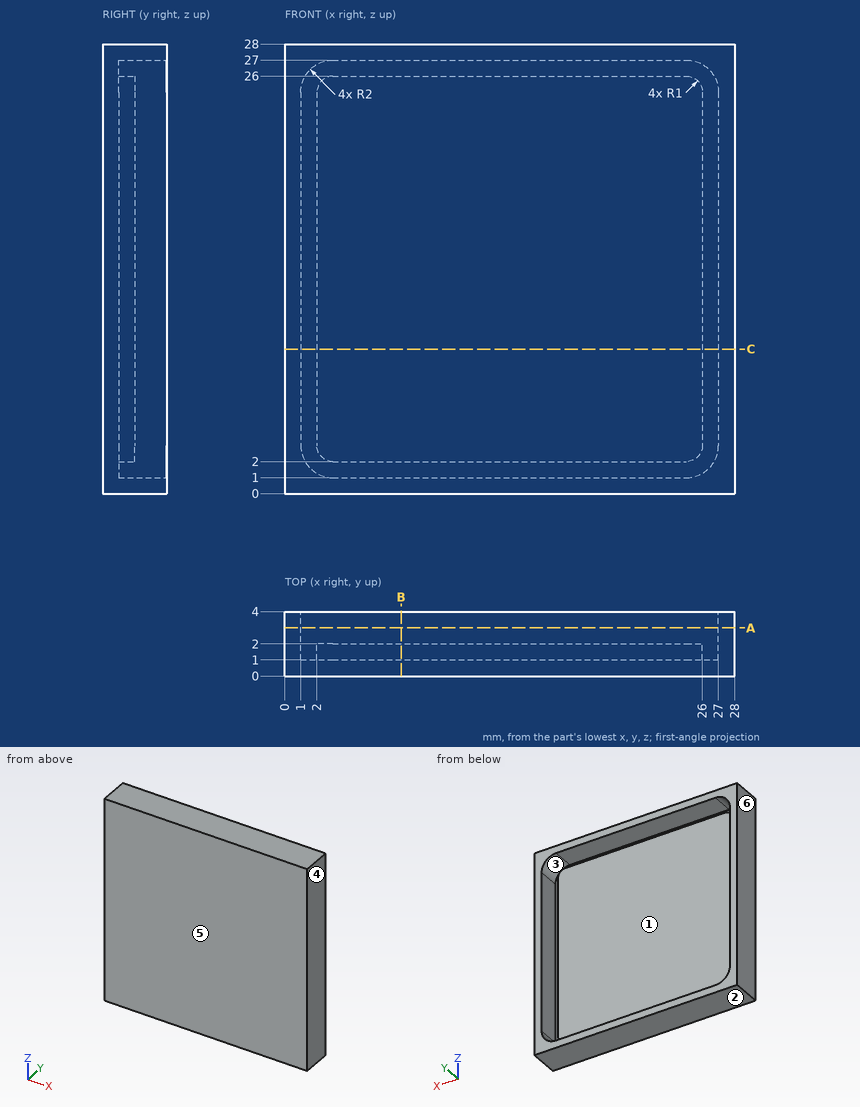
Verification items for this drawing (mm, ordinates from the low corner). A direction names the side the tool comes from. Coordinates: 2 decimals unless noted, no trailing zeros. Order: outer loops, then holes, each group sorted by start corner. A loop starts at its lowest first (then second) coordinate and runs counter-clockwise, first axis right, second up. Notation, with made-up numbers: (74.25, 68.25) - (112.25, 68.25) arc R19 ccw to (112.25, 94.25) - close; hole circle Ø6 at (-6, 2.5). An arc over 180 degrees is marked (long way). Answer in a Markdown table with one row per item. Add a question column.
1. Gauge pin test, flat ends, axial feed: pin 1 Ø1 at (x, z) = (21, 8.5) entering from -Y; pin 2 Ø7 at (x, z) = (13, 10.5) entering from +Y. Record the tip position at first contact, or that the pin passes through.
2. Section check C-C (z = 9). Enter the section's corners in (x, y).
3. Access from +Z, -Z, +X, -X, +Y, -Y to the whole of each face (thin tool, end or side, straight path). Record for the marked faces 1 and 2.
4. Section check B-B (x = 7.25). Enter the section's corners in (y, z).
5. Draft check along X on the marked faces 3, 4, 5 and 6. Enter one of: +X half, -X half, draft (parallel to the pull), parting line (faces both ways), or undercut.
6. Section check A-A (y = 3). Enter the section's corners in (x, z), plus the area to 3 significant figures.
7. Material ranges on L1, parallel to X at y = 1.1, z = 18.5; L2, parallel to X at y = 3.6, z = 12.5, recorded low to high. Write a range as [from, to].
Data:
| question | item | result |
|---|---|---|
| 1 | pin 1 | stops at y = 0 |
| 1 | pin 2 | stops at y = 2 |
| 2 | outline | (0, 0) - (28, 0) - (28, 4) - (27, 4) - (27, 1) - (26, 1) - (26, 2) - (2, 2) - (2, 1) - (1, 1) - (1, 4) - (0, 4) - close |
| 3 | face 1 | +Y |
| 3 | face 2 | -Z, +X, -X, +Y, -Y |
| 4 | outline | (0, 0) - (4, 0) - (4, 1) - (1, 1) - (1, 2) - (2, 2) - (2, 26) - (1, 26) - (1, 27) - (4, 27) - (4, 28) - (0, 28) - close |
| 5 | face 3 | undercut |
| 5 | face 4 | +X half |
| 5 | face 5 | draft |
| 5 | face 6 | -X half |
| 6 | outline | (0, 0) - (28, 0) - (28, 28) - (0, 28) - close; hole (1, 3) arc R2 ccw to (3, 1) - (25, 1) arc R2 ccw to (27, 3) - (27, 25) arc R2 ccw to (25, 27) - (3, 27) arc R2 ccw to (1, 25) - close |
| 6 | area | 111 mm² |
| 7 | L1 | x = [0, 1], [2, 26], [27, 28] |
| 7 | L2 | x = [0, 1], [27, 28] |
